```python
from build123d import *

# Parameters (mm, degrees)
SKETCH_W        = 63
SKETCH_H        = 47
SKETCH_W_2      = 49
SKETCH_H_2      = 23
PAD_DEPTH       = 0.3
SKETCH001_W     = 65
SKETCH001_H     = 49
SKETCH001_W_2   = 63
SKETCH001_H_2   = 47
PAD001_DEPTH    = 6.8
SKETCH002_W     = 4.15
SKETCH002_H     = 4.15
SKETCH002_R     = 1.1
PAD002_DEPTH    = 4.7
SKETCH003_W     = 8.85
SKETCH003_H     = 4.15
SKETCH003_W_2   = 15.85
PAD003_DEPTH    = 4.7
SKETCH004_W     = 37
SKETCH004_H     = 4.15
PAD004_DEPTH    = 1.5
CHAMFER_SIZE    = 1
PAD005_DEPTH    = 0.5
CHAMFER001_SIZE = 1.5
SKETCH006_W     = 80
SKETCH006_H     = 80
SKETCH006_W_2   = 65
SKETCH006_H_2   = 49
PAD006_DEPTH    = 24
SKETCH007_W     = 68
SKETCH007_H     = 68
SKETCH007_W_2   = 65
SKETCH007_H_2   = 49
POCKET_DEPTH    = 17.2
SKETCH008_W     = 14
SKETCH008_H     = 11.2
POCKET001_DEPTH = 6
SKETCH009_W     = 17
SKETCH009_H     = 8
POCKET002_DEPTH = 6
SKETCH010_W     = 26
SKETCH010_H     = 8
PAD007_DEPTH    = 2
CHAMFER002_SIZE = 1.999
SKETCH011_W     = 14
SKETCH011_H     = 1.2
PAD008_DEPTH    = 11.2
SKETCH012_W     = 8.5
SKETCH012_H     = 3
POCKET003_DEPTH = 1.2
SKETCH013_W     = 72.8
SKETCH013_H     = 72.8
SKETCH013_W_2   = 68
SKETCH013_H_2   = 68
PAD009_DEPTH    = 4
FILLET_R        = 9
CHAMFER003_SIZE = 3
CHAMFER004_SIZE = 1
CHAMFER005_SIZE = 1


with BuildPart() as part:
    # Sketch → Pad (new body)
    with BuildSketch(Plane.XY):
        with Locations((0, -1.5)):
            Rectangle(SKETCH_W, SKETCH_H)
        with Locations((0, 1)):
            Rectangle(SKETCH_W_2, SKETCH_H_2, mode=Mode.SUBTRACT)
    extrude(amount=PAD_DEPTH)

    # Sketch001 (on Face10 of Pad) → Pad001 (join)
    with BuildSketch(Plane.XY.offset(0.3)):
        with Locations((0, -1.5)):
            Rectangle(SKETCH001_W, SKETCH001_H)
        with Locations((0, -1.5)):
            Rectangle(SKETCH001_W_2, SKETCH001_H_2, mode=Mode.SUBTRACT)
    extrude(amount=-PAD001_DEPTH)

    # Sketch002 (on Face4 of Pad001) → Pad002 (join)
    with BuildSketch(Plane(origin=(0, 0, 0), x_dir=(1, 0, 0), z_dir=(0, 0, -1))):
        with Locations((-29.425, 22.925)):
            Rectangle(SKETCH002_W, SKETCH002_H)
        with Locations((-29.17, 22.67)):
            Circle(SKETCH002_R, mode=Mode.SUBTRACT)
        with Locations((-29.425, -19.925)):
            Rectangle(SKETCH002_W, SKETCH002_H)
        with Locations((-29.17, -19.67)):
            Circle(SKETCH002_R, mode=Mode.SUBTRACT)
        with Locations((29.425, -19.925)):
            Rectangle(SKETCH002_W, SKETCH002_H)
        with Locations((29.17, -19.67)):
            Circle(SKETCH002_R, mode=Mode.SUBTRACT)
        with Locations((29.425, 22.925)):
            Rectangle(SKETCH002_W, SKETCH002_H)
        with Locations((29.17, 22.67)):
            Circle(SKETCH002_R, mode=Mode.SUBTRACT)
    extrude(amount=PAD002_DEPTH)

    # Sketch003 (on Face4 of Pad002) → Pad003 (join)
    with BuildSketch(Plane(origin=(0, 0, 0), x_dir=(1, 0, 0), z_dir=(0, 0, -1))):
        with Locations((-22.925, -19.925)):
            Rectangle(SKETCH003_W, SKETCH003_H)
        with Locations((22.925, -19.925)):
            Rectangle(SKETCH003_W, SKETCH003_H)
        with Locations((-19.425, 22.925)):
            Rectangle(SKETCH003_W_2, SKETCH003_H)
        with Locations((19.425, 22.925)):
            Rectangle(SKETCH003_W_2, SKETCH003_H)
    extrude(amount=PAD003_DEPTH)

    # Sketch004 (on Face4 of Pad003) → Pad004 (join)
    with BuildSketch(Plane(origin=(0, 0, 0), x_dir=(1, 0, 0), z_dir=(0, 0, -1))):
        with Locations((0, -19.925)):
            Rectangle(SKETCH004_W, SKETCH004_H)
    extrude(amount=PAD004_DEPTH)

    # Chamfer
    chamfer_edges = [part.edges().sort_by_distance(p)[0] for p in [
        (-18.5, 19.925, -1.5),
        (18.5, 19.925, -1.5),
        (-18.5, 19.925, -4.7),
        (18.5, 19.925, -4.7),
    ]]
    chamfer(chamfer_edges, length=CHAMFER_SIZE)

    # Sketch005 (on Face6 of Chamfer) → Pad005 (join)
    with BuildSketch(Plane(origin=(0, 0, 0), x_dir=(1, 0, 0), z_dir=(0, 0, -1))):
        Polygon((11.5, 20.85), (11.5, 25), (-11.5, 25), (-11.5, 20.85), (-31.5, 20.85), (-31.5, 15.85), (31.5, 15.85), (31.5, 20.85), align=None)
    extrude(amount=PAD005_DEPTH)

    # Chamfer001
    chamfer001_edges = [part.edges().sort_by_distance(p)[0] for p in [
        (-11.5, -22.925, -4.7),
        (11.5, -22.925, -4.7),
    ]]
    chamfer(chamfer001_edges, length=CHAMFER001_SIZE)

    # Sketch006 (on Face52 of Chamfer001) → Pad006 (join)
    with BuildSketch(Plane.XY.offset(0.3)):
        Rectangle(SKETCH006_W, SKETCH006_H)
        with Locations((0, -1.5)):
            Rectangle(SKETCH006_W_2, SKETCH006_H_2, mode=Mode.SUBTRACT)
    extrude(amount=-PAD006_DEPTH)

    # Sketch007 (on Face49 of Pad006) → Pocket (cut)
    with BuildSketch(Plane(origin=(0, 0, -23.7), x_dir=(1, 0, 0), z_dir=(0, 0, -1))):
        Rectangle(SKETCH007_W, SKETCH007_H)
        with Locations((0, 1.5)):
            Rectangle(SKETCH007_W_2, SKETCH007_H_2, mode=Mode.SUBTRACT)
    extrude(amount=-POCKET_DEPTH, mode=Mode.SUBTRACT)

    # Sketch008 (on Face49 of Pocket) → Pocket001 (cut)
    with BuildSketch(Plane(origin=(0, -34, 0), x_dir=(-1, 0, 0), z_dir=(0, 1, 0))):
        with Locations((-21, -12.1)):
            Rectangle(SKETCH008_W, SKETCH008_H)
    extrude(amount=-POCKET001_DEPTH, mode=Mode.SUBTRACT)

    # Sketch009 (on Face47 of Pocket001) → Pocket002 (cut)
    with BuildSketch(Plane.XZ.offset(-34)):
        with Locations((-5.5, -13.7)):
            Rectangle(SKETCH009_W, SKETCH009_H)
    extrude(amount=-POCKET002_DEPTH, mode=Mode.SUBTRACT)

    # Sketch010 (on Face24 of Pocket002) → Pad007 (join)
    with BuildSketch(Plane(origin=(0, 0, -6.5), x_dir=(1, 0, 0), z_dir=(0, 0, -1))):
        with Locations((21, 30)):
            Rectangle(SKETCH010_W, SKETCH010_H)
    extrude(amount=PAD007_DEPTH)

    # Chamfer002
    chamfer002_edges = [part.edges().sort_by_distance(p)[0] for p in [
        (21, -26, -8.5),
        (8, -30, -8.5),
    ]]
    chamfer(chamfer002_edges, length=CHAMFER002_SIZE)

    # Sketch011 (on Face55 of Chamfer002) → Pad008 (join)
    with BuildSketch(Plane(origin=(0, 0, -6.5), x_dir=(1, 0, 0), z_dir=(0, 0, -1))):
        with Locations((21, 34.6)):
            Rectangle(SKETCH011_W, SKETCH011_H)
    extrude(amount=PAD008_DEPTH)

    # Sketch012 (on Face17 of Pad008) → Pocket003 (cut)
    with BuildSketch(Plane(origin=(0, -34, 0), x_dir=(-1, 0, 0), z_dir=(0, 1, 0))):
        with Locations((-21, -10)):
            Rectangle(SKETCH012_W, SKETCH012_H)
    extrude(amount=-POCKET003_DEPTH, mode=Mode.SUBTRACT)

    # Sketch013 (on Face15 of Pocket003) → Pad009 (join)
    with BuildSketch(Plane(origin=(0, 0, -23.7), x_dir=(1, 0, 0), z_dir=(0, 0, -1))):
        Rectangle(SKETCH013_W, SKETCH013_H)
        Rectangle(SKETCH013_W_2, SKETCH013_H_2, mode=Mode.SUBTRACT)
    extrude(amount=PAD009_DEPTH)

    # Fillet
    fillet_edges = [part.edges().sort_by_distance(p)[0] for p in [
        (-40, -40, -11.7),
        (40, -40, -11.7),
        (40, 40, -11.7),
        (-40, 40, -11.7),
    ]]
    fillet(fillet_edges, radius=FILLET_R)

    # Chamfer003
    chamfer003_edges = [part.edges().sort_by_distance(p)[0] for p in [
        (36.4, 36.4, -25.7),
        (-36.4, 36.4, -25.7),
        (36.4, -36.4, -25.7),
        (-36.4, -36.4, -25.7),
    ]]
    chamfer(chamfer003_edges, length=CHAMFER003_SIZE)

    # Chamfer004
    chamfer004_edges = [part.edges().sort_by_distance(p)[0] for p in [
        (28, -40, -12.1),
        (21, -40, -17.7),
        (14, -40, -12.1),
        (21, -40, -6.5),
    ]]
    chamfer(chamfer004_edges, length=CHAMFER004_SIZE)

    # Chamfer005
    chamfer005_edges = [part.edges().sort_by_distance(p)[0] for p in [
        (-37.363961, -37.363961, 0.3),
        (-40, 0, 0.3),
        (-37.363961, 37.363961, 0.3),
        (0, 40, 0.3),
        (0, -40, 0.3),
        (37.363961, -37.363961, 0.3),
        (40, 0, 0.3),
        (37.363961, 37.363961, 0.3),
    ]]
    chamfer(chamfer005_edges, length=CHAMFER005_SIZE)


solid = part.part
```
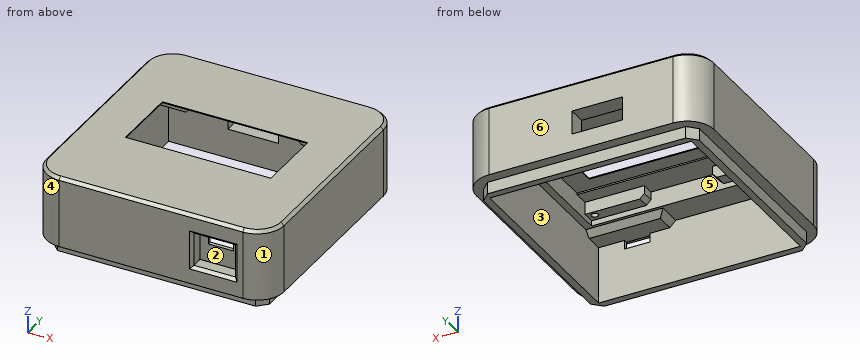
The model under review builds one solid part; all positions refer to its coordinate system, in mm. Face numbers are marked on the shaded views. A direction names the side the tool comes from. Round coordinates to 2 decimals unless told otherwise and drop trailing zeros. Write each loop counter-clockwise with the first axis right and the second up, starting at its lowest first coordinate (ties: lowest second). Pieces come first, ordered by that corner, then holes. Notation, with made-up numbers: M 64.5,-17 L 86.5,-17 A21 cw 86.5,19 Z; hole C 59.5,0 d7. An arc over 180 degrees is marked long. Use CSV: the item, a comma, the result in double quotes. Start each with the question number.
(1) Tool access review of the marked faces 1, 2 and 3: name each direction out of +Z, -Z, +X, -X, +Y, -Y from which nothing blocks a thin tool from reaching the whole face with its end or side.
(2) We need section A-A, the plane x = -15.5. State the section outline as (y, z) points, then the cut area to 3 significant figures.
(3) We need section D-D, the plane y = 3.5. State the section outline as (x, z) points, then the cut area to 3 significant figures.
(4) For line 1 along X through (y, z) = (19.67, -1); line 2 along Y through (x, z) = (29.17, -1.8); line 3 along X through (y, z) = (19.67, -2.85), list the stretches that pass through material, from the lowest coordinate up.
(5) The part is to be moulded in two halves that separate along X. For the marked faces 4, 5 and 6, say which applies: +X half, -X half, draft (parallel to the pull), parting line (faces both ways), or undercut.
(6) Clearance check with flat-ended pins moving along their axes: P1, Ø1.8, axis at y = 38, z = -15, coming from the +X side; P2, Ø2, axis at x = -16.5, y = 15, coming from the -Z side; P3, Ø1.2, axis at y = -5, z = -25.5, coming from the +X side; P4, Ø4, axis at x = 24.5, z = -6.5, coming from the -Y side. State where each tip first meets the part, or that it passes through.
Findings:
1,face 1,"+Z, -Z, +X, -Y"
1,face 2,"-Y"
1,face 3,"-Z"
2,outline,"M -40,-23.7 L -36.4,-23.7 L -36.4,-27.7 L -34,-27.7 L -34,-6.5 L -25,-6.5 L -25,-4.7 L -20.85,-4.7 L -20.85,-0.5 L -15.85,-0.5 L -15.85,0 L -10.5,0 L -10.5,0.3 L -39,0.3 L -40,-0.7 Z; M 12.5,0 L 17.85,0 L 17.85,-1.5 L 22,-1.5 L 22,-6.5 L 34,-6.5 L 34,-27.7 L 36.4,-27.7 L 36.4,-23.7 L 40,-23.7 L 40,-0.7 L 39,0.3 L 12.5,0.3 Z"
2,area,"484 mm^2"
3,outline,"M -40,-23.7 L -36.4,-23.7 L -36.4,-27.7 L -34,-27.7 L -34,-6.5 L -31.5,-6.5 L -31.5,0 L -24.5,0 L -24.5,0.3 L -39,0.3 L -40,-0.7 Z; M 24.5,0 L 31.5,0 L 31.5,-6.5 L 34,-6.5 L 34,-27.7 L 36.4,-27.7 L 36.4,-23.7 L 40,-23.7 L 40,-0.7 L 39,0.3 L 24.5,0.3 Z"
3,area,"344 mm^2"
4,line 1,"-40 to -30.27, -28.07 to 28.07, 30.27 to 40"
4,line 2,"-40 to -23.77, -21.57 to -20.85, 17.85 to 18.57, 20.77 to 40"
4,line 3,"-40 to -30.27, -28.07 to -18.5, 18.5 to 28.07, 30.27 to 40"
5,face 4,"-X half"
5,face 5,"undercut"
5,face 6,"draft"
6,P1,"x = 37.62"
6,P2,"z = 0"
6,P3,"x = 36.4"
6,P4,"y = -40"
